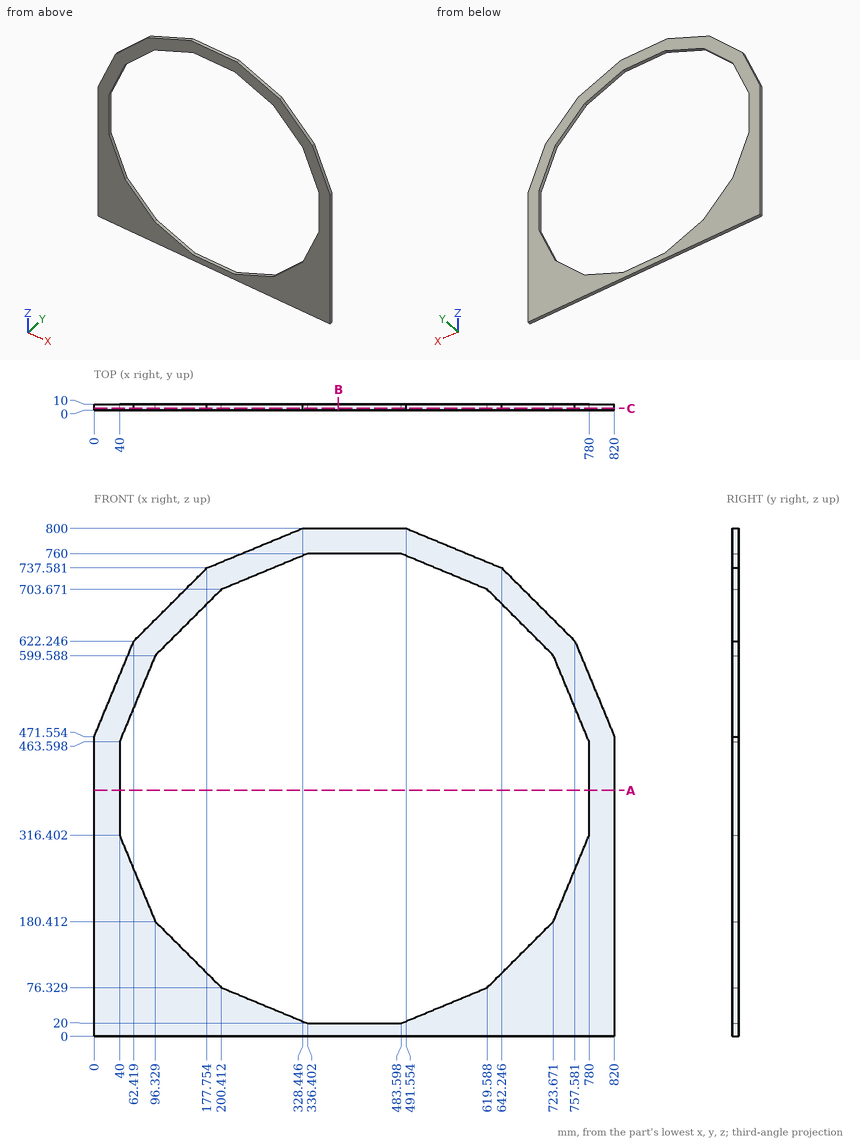
Geometry: see drawing. Coordinates: mm, zero at the bounding-box minimum. Coordinates: 2 decimals unless noted, no trailing zeros. Loops run counter-clockwise (first coordinate to the right, second up) from the corner with the lowest first, then second, coordinate; pieces in that order, holes last. Notation, with made-up numbers: (-10, -15.5) -> (5, -15.5) arc R35 cw to (5, 16.5) -> close; hole circle Ø8 at (27.5, 44). An arc over 180 degrees is marked (long way). Write item = value, one per line. Start each with the question number.
Item 1: Cut plane B-B, the plane x = 385. Return loops of the section in (y, z).
Item 2: Material intervals for line 1 (Z direction, x = 372, y = 4.75); line 2 (Z direction, x = 548, y = 2.5) (1 decimal); line 3 (X direction, y = 7, z = 648.5) (1 decimal), sorted ascending.
Item 3: Cut plane C-C, the plane y = 3. Return loops of the section in (x, z) (1 decimal).
Item 4: Cut plane A-A, the plane z = 387. Return loops of the section in (x, y).
Ans:
q1.outline = (0, 0) -> (10, 0) -> (10, 20) -> (0, 20) -> close; (0, 760) -> (10, 760) -> (10, 800) -> (0, 800) -> close
q2.line_1 = 0 to 20, 760 to 800
q2.line_2 = 0 to 46.7, 733.3 to 776.6
q2.line_3 = 88.7 to 145.2, 674.8 to 731.3
q3.outline = (0, 0) -> (820, 0) -> (820, 471.6) -> (757.6, 622.2) -> (642.2, 737.6) -> (491.6, 800) -> (328.4, 800) -> (177.8, 737.6) -> (62.4, 622.2) -> (0, 471.6) -> close; hole (40, 316.4) -> (96.3, 180.4) -> (200.4, 76.3) -> (336.4, 20) -> (483.6, 20) -> (619.6, 76.3) -> (723.7, 180.4) -> (780, 316.4) -> (780, 463.6) -> (723.7, 599.6) -> (619.6, 703.7) -> (483.6, 760) -> (336.4, 760) -> (200.4, 703.7) -> (96.3, 599.6) -> (40, 463.6) -> close
q4.outline = (0, 0) -> (40, 0) -> (40, 10) -> (0, 10) -> close; (780, 0) -> (820, 0) -> (820, 10) -> (780, 10) -> close
